Geometry check sheet. Reference: the model listing, model coordinates, mm. A direction names the side the tool comes from. Coordinates: 2 decimals unless noted, no trailing zeros. Order: outer loops, then holes, each group sorted by start corner. A loop starts at its lowest first (then second) coordinate and runs counter-clockwise, first axis right, second up. Notation, with made-up numbers: (62.5, 74) - (83.5, 74) arc R28 ccw to (83.5, 104) - close; hole circle Ø5 at (86.25, 7). An arc over 180 degrees is marked (long way). Return JSON: item names as keys, results as strings. Group by question number.
Item 1: Section check B-B on x = -58.5. Enter the section's corners in (y, z), then the cut area to 3 significant figures.
Item 2: Scan lines: probe 1 along Y at (x, z) = (-301.55, -75.75); probe 2 along X at (y, z) = (460, 1.1); probe 3 along Y at (x, z) = (0, 0.75). Record each from-to range of solid material in increasing order.
Item 3: Tool access check on faces 1 (the flat face through (-300.5, 6, -75)), 2 (the flat face through (8, -480, 1)). Record the directions out of +Z, -Z, +X, -X, +Y, -Y that give a thin tool (end or side, any length) a straight path to the whole face; none if there is none.
Item 4: Gauge pin test, flat ends, axial feed: pin 1 (10 mm diameter, centred on y = 339.5, z = -133.5, fed in from +X); pin 2 (13 mm diameter, centred on x = -280.5, y = 460, fed in from -Z); pin 3 (3.5 mm diameter, centred on x = -301, z = -76.5, fed in from -Y); pin 4 (0.9 mm diameter, centred on x = -300, z = -50, fed in from +Y). Record the tip position at first contact, or that the pin passes through.
Item 5: Section check A-A on y = 206. Enter the section's corners in (x, z), then the cut area to 3 significant figures.
Item 6: Draft check along X on faces 3 (the flat face through (4, 7, 0)), 4 (the flat face through (-302, 6, -77)), 5 (the flat face through (8, 480, 1)). Enter one of: pulls with the +X half, pulls with the -X half, needs draft (parallel to the pull), parting line crosses it, or undercut.
from build123d import *

# Parameters (mm, degrees)
BASE_FLANGE1_DEPTH            = 480
CUT_EXTRUDE1_START            = -3
SKETCH6_W                     = 170
SKETCH6_H                     = 41
CUT_EXTRUDE1_DEPTH            = 789.949107767
M5_CLEARANCE_HOLE1_D          = 5.8
FILLET1_R                     = 15
M8_CLEARANCE_HOLE1_AT_2_COUNT = 2
M8_CLEARANCE_HOLE1_AT_2_PITCH = 280.5
M8_CLEARANCE_HOLE1_AT_3_COUNT = 2
M8_CLEARANCE_HOLE1_AT_3_PITCH = 561
M8_CLEARANCE_HOLE2_D          = 10
M8_CLEARANCE_HOLE2_DEPTH      = 8.995696905
M8_CLEARANCE_HOLE2_TIP        = 3.004303095
M8_CLEARANCE_HOLE3_D          = 10
M8_CLEARANCE_HOLE3_DEPTH      = 8.995696905
M8_CLEARANCE_HOLE3_TIP        = 3.004303095


# Sheet-metal steps are written as plain solids
with BuildPart() as part:
    # Sketch1 → Base-Flange1 (new, symmetric)
    with BuildSketch(Plane(origin=(0, 0, 0), x_dir=(1, 0, 0), z_dir=(0, 1, 0))):
        with BuildLine():
            Line((300.5, 40), (300.5, 1.5))
            ThreePointArc((300.5, 1.5), (300.060660172, 0.439339828), (299, 0))
            Line((299, 0), (-299, 0))
            ThreePointArc((-299, 0), (-300.060660172, 0.439339828), (-300.5, 1.5))
            Line((-300.5, 1.5), (-300.5, 150))
            Line((-300.5, 150), (-302, 150))
            Line((-302, 150), (-302, 1.5))
            ThreePointArc((-302, 1.5), (-301.121320344, -0.621320344), (-299, -1.5))
            Line((-299, -1.5), (299, -1.5))
            ThreePointArc((299, -1.5), (301.121320344, -0.621320344), (302, 1.5))
            Line((302, 1.5), (302, 40))
            Line((302, 40), (300.5, 40))
        make_face()
    extrude(amount=BASE_FLANGE1_DEPTH, both=True)

    # Sketch6 → Cut-Extrude1 (cut)
    with BuildSketch(Plane.ZY.offset(302).offset(CUT_EXTRUDE1_START)):
        with Locations((-73.5, 459.5)):
            Rectangle(SKETCH6_W, SKETCH6_H)
    cut_extrude1 = extrude(amount=CUT_EXTRUDE1_DEPTH, mode=Mode.SUBTRACT)

    # Mirror1: Cut-Extrude1 across plane
    add(cut_extrude1.mirror(Plane.ZX), mode=Mode.SUBTRACT)

    # M5 Clearance Hole1 (through all)
    with Locations(Plane.ZY.offset(302)):
        with Locations((-75.75, -379), (-75.75, -189.5), (-75.75, 0), (-75.75, 189.5), (-75.75, 379)):
            Hole(M5_CLEARANCE_HOLE1_D / 2)

    # Fillet1
    fillet1_edges = [part.edges().sort_by_distance(p)[0] for p in [
        (301.25, -480, -40),
        (-299, -480, 0.75),
        (-299, 480, 0.75),
        (301.25, 480, -40),
        (-301.25, 439, -150),
        (-301.25, -439, -150),
    ]]
    fillet(fillet1_edges, radius=FILLET1_R)

    # Sketch10 → M8 Clearance Hole1 (revolve, cut)
    with BuildSketch(Plane(origin=(-280.5, 460, 1.5), x_dir=(0, -1, 0), z_dir=(1, 0, 0))):
        Polygon((0, 0), (0, 12), (5, 8.995696905), (5, 0), align=None)
    m8_clearance_hole1 = revolve(axis=Axis((-280.5, 460, 7.85), (0, 0, -1)), mode=Mode.SUBTRACT)

    # M8 Clearance Hole1 at 2: M8 Clearance Hole1 ×2
    with Locations(*[(i * M8_CLEARANCE_HOLE1_AT_2_PITCH, 0, 0) for i in range(1, M8_CLEARANCE_HOLE1_AT_2_COUNT)]):
        add(m8_clearance_hole1, mode=Mode.SUBTRACT)

    # M8 Clearance Hole1 at 3: M8 Clearance Hole1 ×2
    with Locations(*[(i * M8_CLEARANCE_HOLE1_AT_3_PITCH, 0, 0) for i in range(1, M8_CLEARANCE_HOLE1_AT_3_COUNT)]):
        add(m8_clearance_hole1, mode=Mode.SUBTRACT)

    # Mirror2: M8 Clearance Hole1 across plane
    add(m8_clearance_hole1.mirror(Plane.ZX), mode=Mode.SUBTRACT)

    # Mirror2 copy 1 sketch → Mirror2 copy 1 (revolve, cut)
    with BuildSketch(Plane(origin=(0, -460, 1.5), x_dir=(0, 1, 0), z_dir=(1, 0, 0))):
        Polygon((0, 0), (0, -12), (5, -8.995696905), (5, 0), align=None)
    revolve(axis=Axis((0, -460, 7.85), (0, 0, 1)), mode=Mode.SUBTRACT)

    # Mirror2 copy 2 sketch → Mirror2 copy 2 (revolve, cut)
    with BuildSketch(Plane(origin=(280.5, -460, 1.5), x_dir=(0, 1, 0), z_dir=(1, 0, 0))):
        Polygon((0, 0), (0, -12), (5, -8.995696905), (5, 0), align=None)
    revolve(axis=Axis((280.5, -460, 7.85), (0, 0, 1)), mode=Mode.SUBTRACT)

    # M8 Clearance Hole2
    with Locations(Plane(origin=(302, 0, 0), x_dir=(0, 0, -1), z_dir=(1, 0, 0))):
        with Locations((20, 410), (20, 136.666666667), (20, -136.666666667), (20, -410)):
            Hole(M8_CLEARANCE_HOLE2_D / 2, depth=M8_CLEARANCE_HOLE2_DEPTH)
            with Locations((0, 0, -(M8_CLEARANCE_HOLE2_DEPTH + M8_CLEARANCE_HOLE2_TIP / 2))):  # 118° drill point
                Cone(0, M8_CLEARANCE_HOLE2_D / 2, M8_CLEARANCE_HOLE2_TIP, mode=Mode.SUBTRACT)

    # M8 Clearance Hole3
    with Locations(Plane.ZY.offset(302)):
        with Locations((-20, 369), (-20, 0), (-20, -369)):
            Hole(M8_CLEARANCE_HOLE3_D / 2, depth=M8_CLEARANCE_HOLE3_DEPTH)
            with Locations((0, 0, -(M8_CLEARANCE_HOLE3_DEPTH + M8_CLEARANCE_HOLE3_TIP / 2))):  # 118° drill point
                Cone(0, M8_CLEARANCE_HOLE3_D / 2, M8_CLEARANCE_HOLE3_TIP, mode=Mode.SUBTRACT)


solid = part.part
Computed:
{
 "1": {"outline": "(-480, 0) - (480, 0) - (480, 1.5) - (-480, 1.5) - close", "area": "1,440 mm²"},
 "2": {"probe 1": "y = -439 to -381.9, -376.1 to -192.4, -186.6 to -2.9, 2.9 to 186.6, 192.4 to 376.1, 381.9 to 439", "probe 2": "x = -299 to -285.5, -275.5 to -5, 5 to 275.5, 285.5 to 300.5", "probe 3": "y = -480 to -465, -455 to 455, 465 to 480"},
 "3": {"face 1": "-Z, +Y, -Y", "face 2": "+Z, -Z, +X, -X, -Y"},
 "4": {"pin 1": "stops at x = -300.5", "pin 2": "stops at z = 0", "pin 3": "stops at y = -439", "pin 4": "passes through"},
 "5": {"outline": "(-302, -150) - (-300.5, -150) - (-300.5, -1.5) arc R1.5 cw to (-299, 0) - (299, 0) arc R1.5 cw to (300.5, -1.5) - (300.5, -40) - (302, -40) - (302, -1.5) arc R3 ccw to (299, 1.5) - (-299, 1.5) arc R3 ccw to (-302, -1.5) - close", "area": "1,190 mm²"},
 "6": {"face 3": "undercut", "face 4": "pulls with the -X half", "face 5": "needs draft"}
}
